from build123d import *

# Parameters (mm, degrees)
SKETCH3_W                    = 15.24
SKETCH3_H                    = 7.2
BOSS_EXTRUDE1_DEPTH          = 8.5
SKETCH4_R                    = 0.65
BOSS_EXTRUDE2_DEPTH          = 3.5
CUT_EXTRUDE1_REACH           = 20.877
CUT_EXTRUDE3_DEPTH           = 15.24
SKETCH13_W                   = 1.5
SKETCH13_H                   = 2
CUT_EXTRUDE4_DEPTH           = 2
CUT_EXTRUDE4_DRAFT           = -6
CUT_EXTRUDE4_PROFILE_2_DEPTH = 2
CUT_EXTRUDE4_PROFILE_2_DRAFT = -6
CUT_EXTRUDE4_PROFILE_3_DEPTH = 2
CUT_EXTRUDE4_PROFILE_3_DRAFT = -6
CUT_EXTRUDE4_PROFILE_4_DEPTH = 2
CUT_EXTRUDE4_PROFILE_4_DRAFT = -6
SKETCH14_R                   = 1.5
SKETCH14_R_2                 = 1.4
CUT_EXTRUDE5_DEPTH           = 2
CUT_EXTRUDE6_DEPTH           = 1


with BuildPart() as part:
    # Sketch3 → Boss-Extrude1 (new body)
    with BuildSketch(Plane(origin=(0, 0, 0), x_dir=(1, 0, 0), z_dir=(0, 1, 0))):
        with Locations((7.62, 3.6)):
            Rectangle(SKETCH3_W, SKETCH3_H)
    extrude(amount=BOSS_EXTRUDE1_DEPTH)

    # Sketch4 → Boss-Extrude2 (add)
    with BuildSketch(Plane(origin=(0, 0, 0), x_dir=(-1, 0, 0), z_dir=(0, -1, 0))):
        with Locations(Location((-1.91, 3.6, 0), (0, 0, 90))):
            Circle(SKETCH4_R)
        with Locations(Location((-5.72, 3.6, 0), (0, 0, 90))):
            Circle(SKETCH4_R)
        with Locations(Location((-9.53, 3.6, 0), (0, 0, 90))):
            Circle(SKETCH4_R)
        with Locations(Location((-13.34, 3.6, 0), (0, 0, 90))):
            Circle(SKETCH4_R)
    extrude(amount=BOSS_EXTRUDE2_DEPTH)

    # Cut-Extrude1: up to this face of the body (flat: up to its plane)
    cut_extrude1_end = Plane(part.part.faces().sort_by_distance((15.24, 4.25, -3.6))[0])
    # Sketch5 → Cut-Extrude1 (cut, up to the picked face)
    with BuildSketch(Plane.ZY, mode=Mode.PRIVATE) as cut_extrude1_sk1:
        Polygon((-2.95, -3), (-2.95, -3.5), (-3.35, -3.5), align=None)
    cut_extrude1_tool1 = split(extrude(cut_extrude1_sk1.sketch, amount=-CUT_EXTRUDE1_REACH, mode=Mode.PRIVATE), bisect_by=cut_extrude1_end, keep=Keep.BOTH, mode=Mode.PRIVATE)
    # Sketch5 → Cut-Extrude1 (cut, up to the picked face)
    with BuildSketch(Plane.ZY, mode=Mode.PRIVATE) as cut_extrude1_sk2:
        Polygon((-4.25, -3), (-3.85, -3.5), (-4.25, -3.5), align=None)
    cut_extrude1_tool2 = split(extrude(cut_extrude1_sk2.sketch, amount=-CUT_EXTRUDE1_REACH, mode=Mode.PRIVATE), bisect_by=cut_extrude1_end, keep=Keep.BOTH, mode=Mode.PRIVATE)
    add(cut_extrude1_tool1.solids().sort_by(Axis((0, -3.333333, -3.083333), (1, 0, 0)))[0], mode=Mode.SUBTRACT)
    add(cut_extrude1_tool2.solids().sort_by(Axis((0, -3.333333, -4.116667), (1, 0, 0)))[0], mode=Mode.SUBTRACT)

    # Sketch8 → Cut-Extrude3 (cut)
    with BuildSketch(Plane(origin=(15.24, 0, 0), x_dir=(0, 0, -1), z_dir=(1, 0, 0))):
        Polygon((0, 5.5), (0.537301365, 5.876222466), (1.35, 8.5), (0, 8.5), align=None)
        Polygon((7.2, 6.5), (5.85, 8.5), (7.2, 8.5), align=None)
    extrude(amount=-CUT_EXTRUDE3_DEPTH, mode=Mode.SUBTRACT)


with BuildPart() as cut_extrude4_tool:
    # Sketch13 → Cut-Extrude4 (with draft: the straight prism first)
    with BuildSketch(Plane.XY):
        with Locations((13.34, 2.98672158)):
            Rectangle(SKETCH13_W, SKETCH13_H)
    extrude(amount=-CUT_EXTRUDE4_DEPTH)
    # Cut-Extrude4: the draft: its side faces are tilted about the plane it starts from
    cut_extrude4_sides = [cut_extrude4_tool.faces().sort_by_distance(p)[0] for p in [
        (13.34, 1.98672158, -1),
        (14.09, 2.98672158, -1),
        (13.34, 3.98672158, -1),
        (12.59, 2.98672158, -1),
    ]]
    draft(cut_extrude4_sides, Plane.XY, CUT_EXTRUDE4_DRAFT)


with BuildPart() as part_1:
    add(part.part)

    # Cut-Extrude4: cut by cut_extrude4_tool
    add(cut_extrude4_tool.part, mode=Mode.SUBTRACT)


with BuildPart() as cut_extrude4_profile_2_tool:
    # Sketch13 → Cut-Extrude4 profile 2 (with draft: the straight prism first)
    with BuildSketch(Plane.XY):
        with Locations((9.53, 2.98672158)):
            Rectangle(SKETCH13_W, SKETCH13_H)
    extrude(amount=-CUT_EXTRUDE4_PROFILE_2_DEPTH)
    # Cut-Extrude4 profile 2: the draft: its side faces are tilted about the plane it starts from
    cut_extrude4_profile_2_sides = [cut_extrude4_profile_2_tool.faces().sort_by_distance(p)[0] for p in [
        (9.53, 1.98672158, -1),
        (10.28, 2.98672158, -1),
        (9.53, 3.98672158, -1),
        (8.78, 2.98672158, -1),
    ]]
    draft(cut_extrude4_profile_2_sides, Plane.XY, CUT_EXTRUDE4_PROFILE_2_DRAFT)


with BuildPart() as part_2:
    add(part_1.part)

    # Cut-Extrude4 profile 2: cut by cut_extrude4_profile_2_tool
    add(cut_extrude4_profile_2_tool.part, mode=Mode.SUBTRACT)


with BuildPart() as cut_extrude4_profile_3_tool:
    # Sketch13 → Cut-Extrude4 profile 3 (with draft: the straight prism first)
    with BuildSketch(Plane.XY):
        with Locations((5.72, 2.98672158)):
            Rectangle(SKETCH13_W, SKETCH13_H)
    extrude(amount=-CUT_EXTRUDE4_PROFILE_3_DEPTH)
    # Cut-Extrude4 profile 3: the draft: its side faces are tilted about the plane it starts from
    cut_extrude4_profile_3_sides = [cut_extrude4_profile_3_tool.faces().sort_by_distance(p)[0] for p in [
        (5.72, 1.98672158, -1),
        (6.47, 2.98672158, -1),
        (5.72, 3.98672158, -1),
        (4.97, 2.98672158, -1),
    ]]
    draft(cut_extrude4_profile_3_sides, Plane.XY, CUT_EXTRUDE4_PROFILE_3_DRAFT)


with BuildPart() as part_3:
    add(part_2.part)

    # Cut-Extrude4 profile 3: cut by cut_extrude4_profile_3_tool
    add(cut_extrude4_profile_3_tool.part, mode=Mode.SUBTRACT)


with BuildPart() as cut_extrude4_profile_4_tool:
    # Sketch13 → Cut-Extrude4 profile 4 (with draft: the straight prism first)
    with BuildSketch(Plane.XY):
        with Locations((1.91, 2.98672158)):
            Rectangle(SKETCH13_W, SKETCH13_H)
    extrude(amount=-CUT_EXTRUDE4_PROFILE_4_DEPTH)
    # Cut-Extrude4 profile 4: the draft: its side faces are tilted about the plane it starts from
    cut_extrude4_profile_4_sides = [cut_extrude4_profile_4_tool.faces().sort_by_distance(p)[0] for p in [
        (1.91, 1.98672158, -1),
        (2.66, 2.98672158, -1),
        (1.91, 3.98672158, -1),
        (1.16, 2.98672158, -1),
    ]]
    draft(cut_extrude4_profile_4_sides, Plane.XY, CUT_EXTRUDE4_PROFILE_4_DRAFT)


with BuildPart() as part_4:
    add(part_3.part)

    # Cut-Extrude4 profile 4: cut by cut_extrude4_profile_4_tool
    add(cut_extrude4_profile_4_tool.part, mode=Mode.SUBTRACT)

    # Sketch14 → Cut-Extrude5 (cut)
    # profile 1 of 4: a face of its own
    with BuildSketch(Plane(origin=(0, 8.5, 0), x_dir=(1, 0, 0), z_dir=(0, 1, 0))):
        with Locations(Location((1.91, 3.6, 0), (0, 0, 270))):
            Circle(SKETCH14_R)
        with Locations(Location((1.91, 3.6, 0), (0, 0, 270))):
            Circle(SKETCH14_R_2, mode=Mode.SUBTRACT)
    # profile 2 of 4: a face of its own
    with BuildSketch(Plane(origin=(0, 8.5, 0), x_dir=(1, 0, 0), z_dir=(0, 1, 0))):
        with Locations(Location((5.72, 3.6, 0), (0, 0, 270))):
            Circle(SKETCH14_R)
        with Locations(Location((5.72, 3.6, 0), (0, 0, 270))):
            Circle(SKETCH14_R_2, mode=Mode.SUBTRACT)
    # profile 3 of 4: a face of its own
    with BuildSketch(Plane(origin=(0, 8.5, 0), x_dir=(1, 0, 0), z_dir=(0, 1, 0))):
        with Locations(Location((9.53, 3.6, 0), (0, 0, 270))):
            Circle(SKETCH14_R)
        with Locations(Location((9.53, 3.6, 0), (0, 0, 270))):
            Circle(SKETCH14_R_2, mode=Mode.SUBTRACT)
    # profile 4 of 4: a face of its own
    with BuildSketch(Plane(origin=(0, 8.5, 0), x_dir=(1, 0, 0), z_dir=(0, 1, 0))):
        with Locations(Location((13.34, 3.6, 0), (0, 0, 270))):
            Circle(SKETCH14_R)
        with Locations(Location((13.34, 3.6, 0), (0, 0, 270))):
            Circle(SKETCH14_R_2, mode=Mode.SUBTRACT)
    extrude(amount=-CUT_EXTRUDE5_DEPTH, mode=Mode.SUBTRACT)

    # Sketch15 → Cut-Extrude6 (cut)
    with BuildSketch(Plane(origin=(0, 8.5, 0), x_dir=(1, 0, 0), z_dir=(0, 1, 0))):
        with BuildLine():
            Line((1.102525711, 2.43897232), (3.07102768, 4.407474289))
            ThreePointArc((3.07102768, 4.407474289), (2.91, 4.6), (2.717474289, 4.76102768))
            Line((2.717474289, 4.76102768), (0.74897232, 2.792525711))
            ThreePointArc((0.74897232, 2.792525711), (0.91, 2.6), (1.102525711, 2.43897232))
        make_face()
        with BuildLine():
            Line((8.732738708, 2.449185318), (10.680814682, 4.397261292))
            ThreePointArc((10.680814682, 4.397261292), (10.519949494, 4.589949494), (10.327261292, 4.750814682))
            Line((10.327261292, 4.750814682), (8.379185318, 2.802738708))
            ThreePointArc((8.379185318, 2.802738708), (8.540050506, 2.610050506), (8.732738708, 2.449185318))
        make_face()
        with BuildLine():
            Line((6.870814682, 2.802738708), (4.922738708, 4.750814682))
            ThreePointArc((4.922738708, 4.750814682), (4.730050506, 4.589949494), (4.569185318, 4.397261292))
            Line((4.569185318, 4.397261292), (6.517261292, 2.449185318))
            ThreePointArc((6.517261292, 2.449185318), (6.709949494, 2.610050506), (6.870814682, 2.802738708))
        make_face()
        with BuildLine():
            Line((14.490814682, 2.802738708), (12.542738708, 4.750814682))
            ThreePointArc((12.542738708, 4.750814682), (12.350050506, 4.589949494), (12.189185318, 4.397261292))
            Line((12.189185318, 4.397261292), (14.137261292, 2.449185318))
            ThreePointArc((14.137261292, 2.449185318), (14.329949494, 2.610050506), (14.490814682, 2.802738708))
        make_face()
    extrude(amount=-CUT_EXTRUDE6_DEPTH, mode=Mode.SUBTRACT)


solid = part_4.part
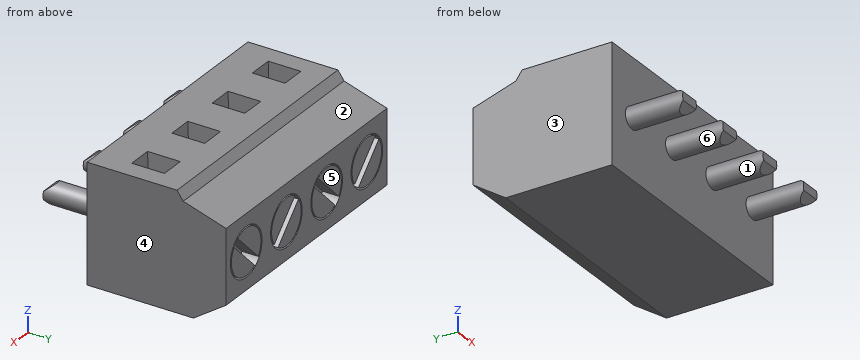
Work out the finished part from the listing and answer in its coordinate system (mm). Face numbers are marked on the shaded views. A direction names the side the tool comes from. Round coordinates to 2 decimals unless told otherwise and drop trailing zeros. Loops run counter-clockwise (first coordinate to the right, second up) from the corner with the lowest first, then second, coordinate; pieces in that order, holes last. Notation, with made-up numbers: (-20, -15.75) - (20, -15.75) arc R17 cw to (20, 2.25) - close; hole circle Ø10 at (42.5, 11.5). An arc over 180 degrees is marked (long way). Use one line per item in the form item = value. Start each with the question number.
(1) Which of the six approach directions +Z, -Z, +X, -X, +Y, -Y give full straight-line access (tool end or side, diameter ignored) to the marked faces 1 and 2?
(2) Determine the mould class of the marked faces 3, 4, 5 and 6 for opening direction X: +X half, -X half, draft (parallel to the pull), parting line (faces both ways), or undercut.
(3) Find section B-B on y = -2.5. Determine the outline of the cut face in (x, z).
(4) Consider line 1 (Z direction, x = 2, y = 2.5); line 2 (Y direction, x = 5, z = -3); line 3 (Z direction, x = 7.75, y = 7.5) (3 decimals). Determine where each line is inside the solid, lowest interval first.
(5) Find section A-A on y = 7.75. Give the number of separate pieces and of enclosed holes in the cut face, and give its area (3 significant figures).
(6) Find section D-D on y = 6.25. Determine the outline of the cut face in (x, z), and give its area (3 significant figures).
(7) Flat-ended cylindrical pins translate along their axes: P1, Ø1, axis at x = 11.5, z = -4.5, coming from the -Y side; P2, Ø1, axis at x = 7, y = 5, coming from the +Z side; P3, Ø1.5, axis at y = -1.5, z = -4, coming from the -X side. Find the tip coordinate at first contact, or state that the pin passes through.
Answer list:
q1.face_1 = -Y
q1.face_2 = +Z, +X, -X, +Y
q2.face_3 = -X half
q2.face_4 = +X half
q2.face_5 = draft
q2.face_6 = undercut
q3.outline = circle Ø1.3 at (1.91, -3.6); circle Ø1.3 at (5.72, -3.6); circle Ø1.3 at (9.53, -3.6); circle Ø1.3 at (13.34, -3.6)
q4.line_1 = -7.2 to -2
q4.line_2 = 0 to 8.5
q4.line_3 = -6.525 to -1.04
q5.separate_pieces = 9
q5.enclosed_holes = 4
q5.area = 70.6 mm^2
q6.outline = (0, -7.2) - (15.24, -7.2) - (15.24, -0.65) - (0, -0.65) - close
q6.area = 99.8 mm^2
q7.P1 = 0
q7.P2 = 0
q7.P3 = 1.26
